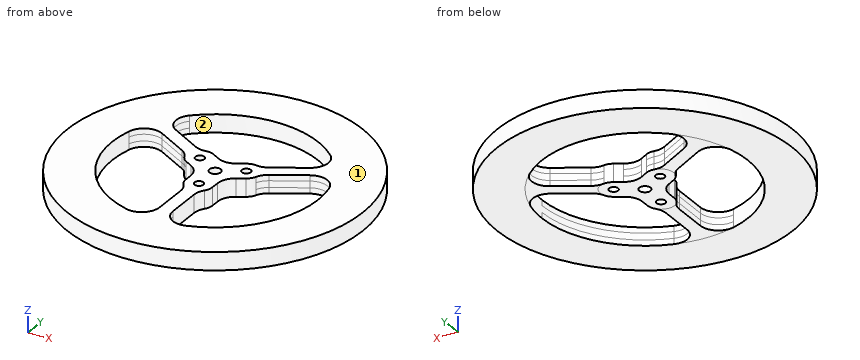
```python
from build123d import *
from build123d.topology import SkipClean

# Parameters (mm, degrees)
BOSS_EXTRUDE1_DEPTH              = 3.175
BOSS_EXTRUDE1_DEPTH_BACK         = 3.175
SKETCH1_R                        = 52.3875
SKETCH1_R_2                      = 2.0193
SHAFT_COUPLER_BOLT_D             = 3.175
SHAFT_COUPLER_BOLT_PATTERN_COUNT = 3
SKETCH6_R                        = 36.5125
CUT_EXTRUDE2_DEPTH               = 2
VOID_CUT_DEPTH                   = 75.214707521
VOID_CUT_DEPTH_BACK              = 75.214707521
TOOLING_RADIUS_R                 = 6.35
BOSS_EXTRUDE2_START              = -4.35
BOSS_EXTRUDE2_DEPTH              = 6.35


# Read off the part's stored shape, not the designer's step: Boss-Extrude2
with BuildPart() as part:
    # Sketch1 → Boss-Extrude1 (new, two sides: drawn at the far end of the back side and taken through both)
    with BuildSketch(Plane.XY.offset(-BOSS_EXTRUDE1_DEPTH_BACK)):
        Circle(SKETCH1_R)
        Circle(SKETCH1_R_2, mode=Mode.SUBTRACT)
    extrude(amount=BOSS_EXTRUDE1_DEPTH + BOSS_EXTRUDE1_DEPTH_BACK)

    # SHAFT-COUPLER-BOLT (through all)
    with Locations(Plane.XY.offset(3.175)):
        with Locations((0, -9.525)):
            shaft_coupler_bolt = Hole(SHAFT_COUPLER_BOLT_D / 2)

    # SHAFT-COUPLER-BOLT-PATTERN: SHAFT-COUPLER-BOLT ×3 about axis
    shaft_coupler_bolt_pattern_axis = Axis((0, 0, 0), (0, 0, 1))
    for i in range(1, SHAFT_COUPLER_BOLT_PATTERN_COUNT):
        add(shaft_coupler_bolt.rotate(shaft_coupler_bolt_pattern_axis, i * 360 / SHAFT_COUPLER_BOLT_PATTERN_COUNT), mode=Mode.SUBTRACT)

    # Sketch6 → Cut-Extrude2 (cut)
    with BuildSketch(Plane.XY.offset(3.175)):
        Circle(SKETCH6_R)
        with BuildLine():
            Line((4.7625, -9.525), (4.7625, -2.749630657))
            Line((4.7625, -2.749630657), (10.630141971, 0.638054014))
            ThreePointArc((10.630141971, 0.638054014), (12.373337957, 7.14375), (5.867641971, 8.886945986))
            Line((5.867641971, 8.886945986), (0, 5.499261314))
            Line((0, 5.499261314), (-5.867641971, 8.886945986))
            ThreePointArc((-5.867641971, 8.886945986), (-12.373337957, 7.14375), (-10.630141971, 0.638054014))
            Line((-10.630141971, 0.638054014), (-4.7625, -2.749630657))
            Line((-4.7625, -2.749630657), (-4.7625, -9.525))
            ThreePointArc((-4.7625, -9.525), (0, -14.2875), (4.7625, -9.525))
        make_face(mode=Mode.SUBTRACT)
    cut_extrude2 = extrude(amount=-CUT_EXTRUDE2_DEPTH, mode=Mode.SUBTRACT)

    # Mirror1: Cut-Extrude2 across plane
    add(cut_extrude2.mirror(Plane.XY), mode=Mode.SUBTRACT)

    # Sketch7 → VOID-CUT (cut, two sides: drawn at the far end of the back side and taken through both)
    with BuildSketch(Plane.XY.offset(1.175).offset(-VOID_CUT_DEPTH_BACK)):
        with BuildLine():
            Line((2.38125, -13.649445986), (2.38125, -36.434767801))
            ThreePointArc((2.38125, -36.434767801), (26.646838901, -24.962143995), (36.5125, 0))
            ThreePointArc((36.5125, 0), (35.557911417, 8.294431382), (32.744059496, 16.155160908))
            Line((32.744059496, 16.155160908), (13.011391971, 4.7625))
            ThreePointArc((13.011391971, 4.7625), (12.373337957, 2.38125), (10.630141971, 0.638054014))
            Line((10.630141971, 0.638054014), (4.7625, -2.749630657))
            Line((4.7625, -2.749630657), (4.7625, -9.525))
            ThreePointArc((4.7625, -9.525), (4.124445986, -11.90625), (2.38125, -13.649445986))
        make_face()
        with BuildLine():
            ThreePointArc((-32.744059496, 16.155160908), (-31.620752556, -18.25625), (-2.38125, -36.434767801))
            Line((-2.38125, -36.434767801), (-2.38125, -13.649445986))
            ThreePointArc((-2.38125, -13.649445986), (-4.124445986, -11.90625), (-4.7625, -9.525))
            Line((-4.7625, -9.525), (-4.7625, -2.749630657))
            Line((-4.7625, -2.749630657), (-10.630141971, 0.638054014))
            ThreePointArc((-10.630141971, 0.638054014), (-12.373337957, 2.38125), (-13.011391971, 4.7625))
            Line((-13.011391971, 4.7625), (-32.744059496, 16.155160908))
        make_face()
        with BuildLine():
            ThreePointArc((30.362809496, 20.279606893), (0, 36.5125), (-30.362809496, 20.279606893))
            Line((-30.362809496, 20.279606893), (-10.630141971, 8.886945986))
            ThreePointArc((-10.630141971, 8.886945986), (-8.248891971, 9.525), (-5.867641971, 8.886945986))
            Line((-5.867641971, 8.886945986), (0, 5.499261314))
            Line((0, 5.499261314), (5.867641971, 8.886945986))
            ThreePointArc((5.867641971, 8.886945986), (8.248891971, 9.525), (10.630141971, 8.886945986))
            Line((10.630141971, 8.886945986), (30.362809496, 20.279606893))
        make_face()
    extrude(amount=VOID_CUT_DEPTH + VOID_CUT_DEPTH_BACK, mode=Mode.SUBTRACT)

    # TOOLING-RADIUS
    # the kernel refuses this fillet: 6.35 mm, written as the material it adds along each edge
    with BuildSketch(Plane(origin=(32.744059496, 16.155160908, 1.175), x_dir=(0.3373763569350217, -0.9413698496240746, 0), z_dir=(0, 0, -1)), Plane(origin=(30.362809496, 20.279606893, -1.175), x_dir=(-0.6465620256636754, 0.7628614205540117, 0), z_dir=(0, 0, 1)), Plane(origin=(-32.744059496, 16.155160908, -1.175), x_dir=(-0.3373763569350221, -0.9413698496240744, 0), z_dir=(0, 0, 1)), Plane(origin=(-2.38125, -36.434767801, 1.175), x_dir=(-0.9839383825986964, 0.17850842907006217, 0), z_dir=(0, 0, -1))) as tooling_radius_piece_1:
        with BuildLine():
            CenterArc((7.598183278, 6.308632991), TOOLING_RADIUS_R, 169.717107938, 106.826448893)
            Line((1.350174548, 7.442161515), (0, 0))
            ThreePointArc((0, 0), (4.16090989, -0.237860303), (8.32181978, 0))
        make_face()
    extrude(amount=2.35)
    with BuildSketch(Plane(origin=(2.38125, -36.434767801, 1.175), x_dir=(0.9839383825986963, 0.17850842907006276, 0), z_dir=(0, 0, -1)), Plane(origin=(-30.362809496, 20.279606893, -1.175), x_dir=(0.6465620256636744, 0.7628614205540126, 0), z_dir=(0, 0, 1))) as tooling_radius_piece_2:
        with BuildLine():
            CenterArc((7.598183278, -6.308632991), TOOLING_RADIUS_R, 83.456443169, 106.826448893)
            Line((1.350174548, -7.442161515), (0, 0))
            ThreePointArc((0, 0), (4.16090989, 0.237860303), (8.32181978, 0))
        make_face()
    extrude(amount=2.35)
    with BuildSketch(Plane(origin=(2.38125, -13.649445986, -1.175), x_dir=(0, -1, 0), z_dir=(0, 0, 1)), Plane(origin=(13.011391971, 4.7625, 1.175), x_dir=(0.866025403784439, 0.4999999999999993, 0), z_dir=(0, 0, -1)), Plane(origin=(-13.011391971, 4.7625, -1.175), x_dir=(-0.8660254037844386, 0.5000000000000001, 0), z_dir=(0, 0, 1)), Plane(origin=(-2.38125, -13.649445986, 1.175), x_dir=(0, -1, 0), z_dir=(0, 0, -1))) as tooling_radius_piece_3:
        with BuildLine():
            CenterArc((2.749630657, 6.35), TOOLING_RADIUS_R, 231.786789298, 38.213210702)
            ThreePointArc((-1.178413139, 1.360714286), (-0.52433438, 0.736538107), (0, 0))
            Line((0, 0), (2.749630657, 0))
        make_face()
    extrude(amount=2.35)
    with BuildSketch(Plane(origin=(10.630141971, 8.886945986, 1.175), x_dir=(0.8660254037844393, 0.4999999999999988, 0), z_dir=(0, 0, -1)), Plane(origin=(-10.630141971, 8.886945986, -1.175), x_dir=(-0.8660254037844384, 0.5000000000000004, 0), z_dir=(0, 0, 1))) as tooling_radius_piece_4:
        with BuildLine():
            CenterArc((2.749630657, -6.35), TOOLING_RADIUS_R, 90, 38.213210702)
            ThreePointArc((-1.178413139, -1.360714286), (-0.52433438, -0.736538107), (0, 0))
            Line((0, 0), (2.749630657, 0))
        make_face()
    extrude(amount=2.35)
    with BuildSketch(Plane(origin=(-4.7625, -2.749630657, -1.175), x_dir=(-0.8660254037844364, 0.5000000000000039, 0), z_dir=(0, 0, 1)), Plane(origin=(4.7625, -2.749630657, -1.175), x_dir=(0, -1, 0), z_dir=(0, 0, 1))) as tooling_radius_piece_5:
        with BuildLine():
            CenterArc((TOOLING_RADIUS_R * 0.57735026919, TOOLING_RADIUS_R), TOOLING_RADIUS_R, 210, 60)
            Line((-TOOLING_RADIUS_R * 0.288675134595, TOOLING_RADIUS_R * 0.5), (0, 0))
            Line((0, 0), (TOOLING_RADIUS_R * 0.57735026919, 0))
        make_face()
    extrude(amount=2.35)
    with BuildSketch(Plane(origin=(0, 5.499261314, 1.175), x_dir=(0.8660254037844363, 0.5000000000000041, 0), z_dir=(0, 0, -1))) as tooling_radius_piece_6:
        with BuildLine():
            CenterArc((TOOLING_RADIUS_R * 0.57735026919, -TOOLING_RADIUS_R), TOOLING_RADIUS_R, 90, 60)
            Line((-TOOLING_RADIUS_R * 0.288675134595, -TOOLING_RADIUS_R * 0.5), (0, 0))
            Line((0, 0), (TOOLING_RADIUS_R * 0.57735026919, 0))
        make_face()
    extrude(amount=2.35)
    with BuildSketch(Plane(origin=(4.7625, -2.749630657, -3.175), x_dir=(0.8660254037844362, 0.5000000000000043, 0), z_dir=(0, 0, 1)), Plane(origin=(0, 5.499261314, -3.175), x_dir=(-0.8660254037844383, 0.5000000000000009, 0), z_dir=(0, 0, 1)), Plane(origin=(-4.7625, -2.749630657, -3.175), x_dir=(0, -1, 0), z_dir=(0, 0, 1))) as tooling_radius_piece_7:
        with BuildLine():
            CenterArc((TOOLING_RADIUS_R * 0.57735026919, -TOOLING_RADIUS_R), TOOLING_RADIUS_R, 90, 60)
            Line((-TOOLING_RADIUS_R * 0.288675134595, -TOOLING_RADIUS_R * 0.5), (0, 0))
            Line((0, 0), (TOOLING_RADIUS_R * 0.57735026919, 0))
        make_face()
    extrude(amount=2)
    with BuildSketch(Plane(origin=(4.7625, -2.749630657, 3.175), x_dir=(0.8660254037844362, 0.5000000000000043, 0), z_dir=(0, 0, -1)), Plane(origin=(0, 5.499261314, 3.175), x_dir=(-0.8660254037844383, 0.5000000000000009, 0), z_dir=(0, 0, -1)), Plane(origin=(-4.7625, -2.749630657, 3.175), x_dir=(0, -1, 0), z_dir=(0, 0, -1))) as tooling_radius_piece_8:
        with BuildLine():
            CenterArc((TOOLING_RADIUS_R * 0.57735026919, TOOLING_RADIUS_R), TOOLING_RADIUS_R, 210, 60)
            Line((-TOOLING_RADIUS_R * 0.288675134595, TOOLING_RADIUS_R * 0.5), (0, 0))
            Line((0, 0), (TOOLING_RADIUS_R * 0.57735026919, 0))
        make_face()
    extrude(amount=2)

    # Boss-Extrude2 outline → Boss-Extrude2 (add)
    with SkipClean():  # the faces are left unmerged after this step: merging them gives an invalid solid
        with BuildSketch(Plane(origin=(0, 0, -1.175), x_dir=(-1, 0, 0), z_dir=(0, 0, -1)).offset(BOSS_EXTRUDE2_START)):
            with BuildLine():
                ThreePointArc((-3.741964286, -12.471032847), (-2.731063991, -14.320551238), (-2.38125, -16.399076643))
                Line((-2.38125, -16.399076643), (-2.38125, -28.871121899))
                ThreePointArc((-2.38125, -28.871121899), (-4.94639879, -33.969886584), (-10.569407895, -34.949252825))
                ThreePointArc((-10.569407895, -34.949252825), (0, -36.5125), (10.569407895, -34.949252825))
                ThreePointArc((10.569407895, -34.949252825), (4.94639879, -33.969886584), (2.38125, -28.871121899))
                Line((2.38125, -28.871121899), (2.38125, -16.399076643))
                ThreePointArc((2.38125, -16.399076643), (2.731063991, -14.320551238), (3.741964286, -12.471032847))
                ThreePointArc((3.741964286, -12.471032847), (0, -14.2875), (-3.741964286, -12.471032847))
            make_face()
            with BuildLine():
                ThreePointArc((-24.982236842, 26.628002152), (-31.620752556, 18.25625), (-35.551644737, 8.321250673))
                ThreePointArc((-35.551644737, 8.321250673), (-31.89198414, 12.701236283), (-26.19375, 12.373337957))
                Line((-26.19375, 12.373337957), (-15.392641971, 6.137315329))
                ThreePointArc((-15.392641971, 6.137315329), (-13.767493164, 4.795104823), (-12.6712134, 2.994880292))
                ThreePointArc((-12.6712134, 2.994880292), (-12.373337957, 7.14375), (-8.929249114, 9.476152555))
                ThreePointArc((-8.929249114, 9.476152555), (-11.036429173, 9.525446415), (-13.011391971, 10.261761314))
                Line((-13.011391971, 10.261761314), (-23.8125, 16.497783942))
                ThreePointArc((-23.8125, 16.497783942), (-26.945585351, 21.268650301), (-24.982236842, 26.628002152))
            make_face()
            with BuildLine():
                ThreePointArc((35.551644737, 8.321250673), (31.620752556, 18.25625), (24.982236842, 26.628002152))
                ThreePointArc((24.982236842, 26.628002152), (26.945585351, 21.268650301), (23.8125, 16.497783942))
                Line((23.8125, 16.497783942), (13.011391971, 10.261761314))
                ThreePointArc((13.011391971, 10.261761314), (11.036429173, 9.525446415), (8.929249114, 9.476152555))
                ThreePointArc((8.929249114, 9.476152555), (12.373337957, 7.14375), (12.6712134, 2.994880292))
                ThreePointArc((12.6712134, 2.994880292), (13.767493164, 4.795104823), (15.392641971, 6.137315329))
                Line((15.392641971, 6.137315329), (26.19375, 12.373337957))
                ThreePointArc((26.19375, 12.373337957), (31.89198414, 12.701236283), (35.551644737, 8.321250673))
            make_face()
        extrude(amount=BOSS_EXTRUDE2_DEPTH)
    add(part.part.scale(1), mode=Mode.REPLACE)  # the faces are merged on a copy


solid = part.part
```
Here's how the part is built. I have some questions about the finished solid (model axes, mm). Face numbers are marked on the shaded views. A direction names the side the tool comes from. Give positions to 0.01 mm unless a question says otherwise; leave off trailing zeros. Order: outer loops, then holes, each group sorted by start corner. A loop starts at its lowest first (then second) coordinate and runs counter-clockwise, first axis right, second up. Notation, with made-up numbers: (2, -32) - (36, -32) arc R24 cw to (36, 1) - close; hole circle Ø7 at (33, 85). An arc over 180 degrees is marked (long way). Answer as a JSON object with one key per item and string values. Group by question number.
Item 1: If we section it at D-D on y = -43: Please give me the cut outline in (x, z) (3 decimals).
Item 2: For P1, Ø1.9, axis at x = 0, y = -9.525, coming from the -Z side; P2, Ø3, axis at y = -9, z = 1.5, coming from the +X side; P3, Ø1.5, axis at y = -33.5, z = -2, coming from the +X side; P4, Ø0.7, axis at y = -23, z = 0, coming from the -X side, each with a flat end and sliding along its axis, tell me the tip position at first contact or that it passes through.
Item 3: Please list where these lines run through material, in increasing order: probe 1 along Y at (x, z) = (0, 1.5); probe 2 along Y at (x, z) = (22.5, -1.75); probe 3 along Y at (x, z) = (8, 1.75).
Item 4: If we section it at B-B on x = 0: Please give me the cut outline in (y, z) (1 decimal), and give its area (3 significant figures).
Item 5: If we section it at C-C on z = 0: Give the number of separate pieces and of enclosed holes in the cut face, and give its area (3 significant figures).
Item 6: Which directions (+Z, -Z, +X, -X, +Y, -Y) give clear straight access to the entire face, cutting with the end or side of a thin tool? Please do the marked faces 1 and 2.
Item 7: If we section it at A-A on x = 19.5: Please give me the cut outline in (y, z) (3 decimals).
Result set:
{
 "1": {"outline": "(-29.924, -3.175) - (29.924, -3.175) - (29.924, 3.175) - (-29.924, 3.175) - close"},
 "2": {"P1": "through", "P2": "x = 51.85", "P3": "x = 40.89", "P4": "x = -47.24"},
 "3": {"probe 1": "-52.39 to -11.11, -7.94 to -2.02, 2.02 to 6.48, 36.51 to 52.39", "probe 2": "-47.31 to -28.76, 10.24 to 15.74, 28.76 to 47.31", "probe 3": "-51.77 to -35.18, -0.88 to 3.19, 6.33 to 9.52, 35.63 to 51.77"},
 "4": {"outline": "(-52.4, -3.2) - (-11.1, -3.2) - (-11.1, 3.2) - (-52.4, 3.2) - close; (-7.9, -3.2) - (-2, -3.2) - (-2, 3.2) - (-7.9, 3.2) - close; (2, -3.2) - (6.5, -3.2) - (6.5, 3.2) - (2, 3.2) - close; (36.5, -3.2) - (52.4, -3.2) - (52.4, 3.2) - (36.5, 3.2) - close", "area": "429 mm²"},
 "5": {"separate pieces": "1", "enclosed holes": "7", "area": "5,150 mm²"},
 "6": {"face 1": "+Z, +X, -X, +Y, -Y", "face 2": "+Z, -Z"},
 "7": {"outline": "(-48.623, -3.175) - (-30.869, -3.175) - (-30.869, 3.175) - (-48.623, 3.175) - close; (8.509, -3.175) - (14.008, -3.175) - (14.008, 3.175) - (8.509, 3.175) - close; (30.869, -3.175) - (48.623, -3.175) - (48.623, 3.175) - (30.869, 3.175) - close"}
}
